Here's how the part is built. I have some questions about the finished solid (model axes, mm). Face numbers are marked on the shaded views. Round coordinates to 2 decimals unless told otherwise and drop trailing zeros. Order: outer loops, then holes, each group sorted by start corner. A loop starts at its lowest first (then second) coordinate and runs counter-clockwise, first axis right, second up.
Autodesk Inventor part; units mm, degrees
ref_plane "YZ Plane" through (0, 0, 0) normal (1, 0, 0) x (0, 1, 0)
ref_plane "XZ Plane" through (0, 0, 0) normal (0, 1, 0) x (-1, 0, 0)
ref_plane "XY Plane" through (0, 0, 0) normal (0, 0, 1) x (1, 0, 0)
sketch "Sketch2" plane through (0, 0, 0) normal (0, 1, 0) x (-1, 0, 0)
  line L0 (0, 0) -> (22, 0)
  line L1 (22, 0) -> (22, -27.18)
  line L2 (22, -27.18) -> (0, -27.18)
  line L3 (0, -27.18) -> (0, 0)
  dimension "d0" = 27.18
  dimension "d1" = 22
extrude "Extrusion1" add sketch "Sketch2" along normal blind 2
sketch "Sketch3" plane through (0, 2, 0) normal (0, 1, 0) x (1, 0, 0)
  line L0 (-22, 0) -> (0, 0)
  line L1 (0, 0) -> (0, 27.18)
  line L2 (0, 27.18) -> (-22, 27.18)
  line L3 (-22, 27.18) -> (-22, 0)
  line L4 (-22, 0) -> (0, 0)
  line L5 (0, 0) -> (0, 27.18)
  line L6 (-22, 0) -> (0, 0)
  line L7 (0, 0) -> (0, 1.5)
  line L8 (0, 1.5) -> (-22, 1.5)
  line L9 (-22, 1.5) -> (-22, 0)
  line L10 (-22, 3.2) -> (0, 3.2)
  line L11 (0, 3.2) -> (0, 4.7)
  line L12 (0, 4.7) -> (-22, 4.7)
  line L13 (-22, 4.7) -> (-22, 3.2)
  line L14 (-22, 6.4) -> (0, 6.4)
  line L15 (0, 6.4) -> (0, 7.9)
  line L16 (0, 7.9) -> (-22, 7.9)
  line L17 (-22, 7.9) -> (-22, 6.4)
  line L18 (-22, 9.6) -> (0, 9.6)
  line L19 (0, 9.6) -> (0, 11.1)
  line L20 (0, 11.1) -> (-22, 11.1)
  line L21 (-22, 11.1) -> (-22, 9.6)
  line L22 (-22, 12.8) -> (0, 12.8)
  line L23 (0, 12.8) -> (0, 14.3)
  line L24 (0, 14.3) -> (-22, 14.3)
  line L25 (-22, 14.3) -> (-22, 12.8)
  line L26 (-22, 16) -> (0, 16)
  line L27 (0, 16) -> (0, 17.5)
  line L28 (0, 17.5) -> (-22, 17.5)
  line L29 (-22, 17.5) -> (-22, 16)
  line L30 (-22, 19.2) -> (0, 19.2)
  line L31 (0, 19.2) -> (0, 20.7)
  line L32 (0, 20.7) -> (-22, 20.7)
  line L33 (-22, 20.7) -> (-22, 19.2)
  line L34 (-22, 22.4) -> (0, 22.4)
  line L35 (0, 22.4) -> (0, 23.9)
  line L36 (0, 23.9) -> (-22, 23.9)
  line L37 (-22, 23.9) -> (-22, 22.4)
  line L38 (-22, 27.18) -> (-22, 0)
  line L39 (0, 27.18) -> (-22, 27.18)
  line L40 (-22, 27.18) -> (-22, 25.68)
  line L41 (-22, 25.68) -> (0, 25.68)
  line L42 (0, 25.68) -> (0, 27.18)
  dimension "d4" = 1.5
  dimension "d7" = 3.2
  dimension "d12" = 1.5
extrude "Extrusion2" add sketch "Sketch3" along normal blind 10 contours L3 L8 L1 L0 | L3 L12 L1 L10 | L3 L16 L1 L14 | L3 L20 L1 L18 | L3 L24 L1 L22 | L3 L28 L1 L26 | L3 L32 L1 L30 | L3 L36 L1 L34 | L3 L2 L1 L41
sketch "Sketch4" plane through (0, 0, 0) normal (0, -1, 0) x (1, 0, 0)
  circle A0 centre (0, -14) radius 4
  line L0 (0, -27.18) -> (0, 0)
  dimension "d15" = 8
  dimension "d16" = 14
extrude "Extrusion3" cut sketch "Sketch4" against normal through all
properties part number "Heatsink" material "Aluminum 6061"
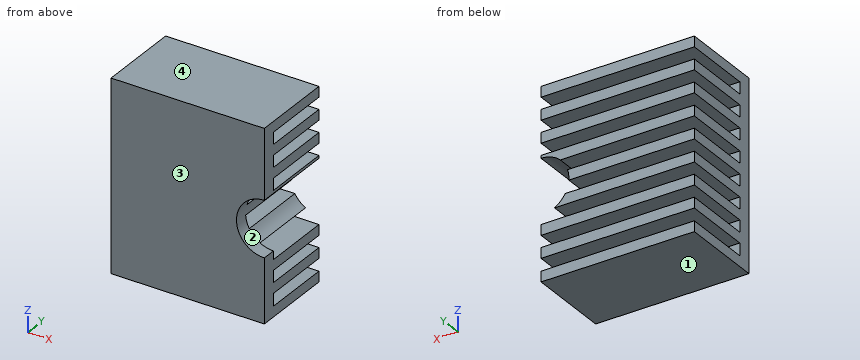
1. I need wall thicknesses on probe 1 along Y at (x, z) = (-2.25, -24); probe 2 along X at (y, z) = (1, -11.75); probe 3 along X at (y, z) = (1, -12.25). Which ranges of each line are inside material? Lowest first, please.
Evaluation:
probe 1: y = 0 to 2
probe 2: x = -22 to -3.31
probe 3: x = -22 to -3.6
2. If we section it at C-C, the plane y = 5.25: State how many separate pieces and enclosed holes the cut face has, and give its area (3 significant figures).
Evaluation:
separate pieces: 9
enclosed holes: 0
area: 285 mm2
3. If we section it at B-B, the plane z = -2: Write out the boundary of the cut face in (x, y), and give its area (3 significant figures).
Evaluation:
outline: (-22, 0) - (0, 0) - (0, 2) - (-22, 2) - close
area: 44.0 mm2
4. If we mould it in two halves opening along Z, with no side actions, what happens to the marked faces 1, 2, 3 and 4? For each: released by +Z, released by -Z, zero draft, split by the parting line, or undercut.
Evaluation:
face 1: released by -Z
face 2: undercut
face 3: zero draft
face 4: released by +Z
5. I'm going to push flat-ended pins straight in: P1, Ø3, axis at x = -6, y = 6, coming from the +Z side; P2, Ø1.4, axis at x = -15.5, z = -12, coming from the +Y side. Where does each tip first touch, or does it pass through?
Evaluation:
P1: stops at z = 0
P2: stops at y = 2
6. If we section it at D-D, the plane z = -14: Write out the boundary of the cut face in (x, y), and give its area (3 significant figures).
Evaluation:
outline: (-22, 0) - (-4, 0) - (-4, 12) - (-22, 12) - close
area: 216 mm2
